For this review, take the finished solid that the model builds, in its own axes (mm). Round coordinates to 2 decimals unless told otherwise and drop trailing zeros. Write each loop counter-clockwise with the first axis right and the second up, starting at its lowest first coordinate (ties: lowest second). Pieces come first, ordered by that corner, then holes. Notation, with made-up numbers: M 6,-11.5 L 35,-11.5 A31 ccw 35,18.5 Z; hole C -28,-7.75 d1. An arc over 180 degrees is marked long. Answer in a Markdown table with one row per item.
```python
from build123d import *

# Parameters (mm, degrees)
SALIENTE_EXTRUIR1_DEPTH = 1
CROQUIS2_R              = 10
CORTAR_EXTRUIR1_DEPTH   = 57.577380639
CROQUIS3_R              = 1.5
CROQUIS3_R_2            = 2.5
CORTAR_EXTRUIR2_DEPTH   = 57.577380639
MATRIZC1_COUNT          = 4


with BuildPart() as part:
    # Croquis1 → Saliente-Extruir1 (new body)
    with BuildSketch(Plane.XY):
        with BuildLine():
            Line((-35, -40), (35, -40))
            ThreePointArc((35, -40), (38.535533906, -38.535533906), (40, -35))
            Line((40, -35), (40, 35))
            ThreePointArc((40, 35), (38.535533906, 38.535533906), (35, 40))
            Line((35, 40), (-35, 40))
            ThreePointArc((-35, 40), (-38.535533906, 38.535533906), (-40, 35))
            Line((-40, 35), (-40, -35))
            ThreePointArc((-40, -35), (-38.535533906, -38.535533906), (-35, -40))
        make_face()
    extrude(amount=SALIENTE_EXTRUIR1_DEPTH)

    # Croquis2 → Cortar-Extruir1 (cut, through all)
    with BuildSketch(Plane.XY.offset(1)):
        Circle(CROQUIS2_R)
        with BuildLine():
            Line((2.5, 16.770509831), (2.5, 30))
            ThreePointArc((2.5, 30), (3.232233047, 31.767766953), (5, 32.5))
            Line((5, 32.5), (22.928932188, 32.5))
            ThreePointArc((22.928932188, 32.5), (25.238631019, 30.956708581), (24.696699141, 28.232233047))
            Line((24.696699141, 28.232233047), (10.090774273, 13.626308179))
            ThreePointArc((10.090774273, 13.626308179), (8.683931275, 12.920265539), (7.134006274, 13.194921541))
            ThreePointArc((7.134006274, 13.194921541), (5.740251485, 13.858192988), (4.285714286, 14.374722712))
            ThreePointArc((4.285714286, 14.374722712), (2.995540686, 15.27647407), (2.5, 16.770509831))
        make_face()
        with BuildLine():
            Line((-10.090774273, 13.626308179), (-24.696699141, 28.232233047))
            ThreePointArc((-24.696699141, 28.232233047), (-25.238631019, 30.956708581), (-22.928932188, 32.5))
            Line((-22.928932188, 32.5), (-5, 32.5))
            ThreePointArc((-5, 32.5), (-3.232233047, 31.767766953), (-2.5, 30))
            Line((-2.5, 30), (-2.5, 16.770509831))
            ThreePointArc((-2.5, 16.770509831), (-2.995540686, 15.27647407), (-4.285714286, 14.374722712))
            ThreePointArc((-4.285714286, 14.374722712), (-5.740251485, 13.858192988), (-7.134006274, 13.194921541))
            ThreePointArc((-7.134006274, 13.194921541), (-8.683931275, 12.920265539), (-10.090774273, 13.626308179))
        make_face()
        with BuildLine():
            Line((32.5, 5), (32.5, 22.928932188))
            ThreePointArc((32.5, 22.928932188), (30.956708581, 25.238631019), (28.232233047, 24.696699141))
            Line((28.232233047, 24.696699141), (13.626308179, 10.090774273))
            ThreePointArc((13.626308179, 10.090774273), (12.920265539, 8.683931275), (13.194921541, 7.134006274))
            ThreePointArc((13.194921541, 7.134006274), (13.858192988, 5.740251485), (14.374722712, 4.285714286))
            ThreePointArc((14.374722712, 4.285714286), (15.27647407, 2.995540686), (16.770509831, 2.5))
            Line((16.770509831, 2.5), (30, 2.5))
            ThreePointArc((30, 2.5), (31.767766953, 3.232233047), (32.5, 5))
        make_face()
        with BuildLine():
            Line((16.770509831, -2.5), (30, -2.5))
            ThreePointArc((30, -2.5), (31.767766953, -3.232233047), (32.5, -5))
            Line((32.5, -5), (32.5, -22.928932188))
            ThreePointArc((32.5, -22.928932188), (30.956708581, -25.238631019), (28.232233047, -24.696699141))
            Line((28.232233047, -24.696699141), (13.626308179, -10.090774273))
            ThreePointArc((13.626308179, -10.090774273), (12.920265539, -8.683931275), (13.194921541, -7.134006274))
            ThreePointArc((13.194921541, -7.134006274), (13.858192988, -5.740251485), (14.374722712, -4.285714286))
            ThreePointArc((14.374722712, -4.285714286), (15.27647407, -2.995540686), (16.770509831, -2.5))
        make_face()
        with BuildLine():
            Line((5, -32.5), (22.928932188, -32.5))
            ThreePointArc((22.928932188, -32.5), (25.238631019, -30.956708581), (24.696699141, -28.232233047))
            Line((24.696699141, -28.232233047), (10.090774273, -13.626308179))
            ThreePointArc((10.090774273, -13.626308179), (8.683931275, -12.920265539), (7.134006274, -13.194921541))
            ThreePointArc((7.134006274, -13.194921541), (5.740251485, -13.858192988), (4.285714286, -14.374722712))
            ThreePointArc((4.285714286, -14.374722712), (2.995540686, -15.27647407), (2.5, -16.770509831))
            Line((2.5, -16.770509831), (2.5, -30))
            ThreePointArc((2.5, -30), (3.232233047, -31.767766953), (5, -32.5))
        make_face()
        with BuildLine():
            Line((-2.5, -16.770509831), (-2.5, -30))
            ThreePointArc((-2.5, -30), (-3.232233047, -31.767766953), (-5, -32.5))
            Line((-5, -32.5), (-22.928932188, -32.5))
            ThreePointArc((-22.928932188, -32.5), (-25.238631019, -30.956708581), (-24.696699141, -28.232233047))
            Line((-24.696699141, -28.232233047), (-10.090774273, -13.626308179))
            ThreePointArc((-10.090774273, -13.626308179), (-8.683931275, -12.920265539), (-7.134006274, -13.194921541))
            ThreePointArc((-7.134006274, -13.194921541), (-5.740251485, -13.858192988), (-4.285714286, -14.374722712))
            ThreePointArc((-4.285714286, -14.374722712), (-2.995540686, -15.27647407), (-2.5, -16.770509831))
        make_face()
        with BuildLine():
            Line((-32.5, -5), (-32.5, -22.928932188))
            ThreePointArc((-32.5, -22.928932188), (-30.956708581, -25.238631019), (-28.232233047, -24.696699141))
            Line((-28.232233047, -24.696699141), (-13.626308179, -10.090774273))
            ThreePointArc((-13.626308179, -10.090774273), (-12.920265539, -8.683931275), (-13.194921541, -7.134006274))
            ThreePointArc((-13.194921541, -7.134006274), (-13.858192988, -5.740251485), (-14.374722712, -4.285714286))
            ThreePointArc((-14.374722712, -4.285714286), (-15.27647407, -2.995540686), (-16.770509831, -2.5))
            Line((-16.770509831, -2.5), (-30, -2.5))
            ThreePointArc((-30, -2.5), (-31.767766953, -3.232233047), (-32.5, -5))
        make_face()
        with BuildLine():
            Line((-16.770509831, 2.5), (-30, 2.5))
            ThreePointArc((-30, 2.5), (-31.767766953, 3.232233047), (-32.5, 5))
            Line((-32.5, 5), (-32.5, 22.928932188))
            ThreePointArc((-32.5, 22.928932188), (-30.956708581, 25.238631019), (-28.232233047, 24.696699141))
            Line((-28.232233047, 24.696699141), (-13.626308179, 10.090774273))
            ThreePointArc((-13.626308179, 10.090774273), (-12.920265539, 8.683931275), (-13.194921541, 7.134006274))
            ThreePointArc((-13.194921541, 7.134006274), (-13.858192988, 5.740251485), (-14.374722712, 4.285714286))
            ThreePointArc((-14.374722712, 4.285714286), (-15.27647407, 2.995540686), (-16.770509831, 2.5))
        make_face()
    extrude(amount=-CORTAR_EXTRUIR1_DEPTH, mode=Mode.SUBTRACT)

    # Croquis3 → Cortar-Extruir2 (cut, through all)
    with BuildSketch(Plane.XY.offset(1)):
        with Locations((-36.25, 30)):
            Circle(CROQUIS3_R)
        with Locations((-36.25, 10)):
            Circle(CROQUIS3_R)
        with Locations((-36.25, -10)):
            Circle(CROQUIS3_R)
        with Locations((-36.25, -30)):
            Circle(CROQUIS3_R)
        with Locations(Location((36.25, -30, 0), (0, 0, 180))):
            Circle(CROQUIS3_R)
        with Locations(Location((36.25, -10, 0), (0, 0, 180))):
            Circle(CROQUIS3_R)
        with Locations(Location((36.25, 10, 0), (0, 0, 180))):
            Circle(CROQUIS3_R)
        with Locations(Location((36.25, 30, 0), (0, 0, 180))):
            Circle(CROQUIS3_R)
        with Locations((-36.25, 0)):
            Circle(CROQUIS3_R_2)
        with Locations(Location((36.25, 0, 0), (0, 0, 180))):
            Circle(CROQUIS3_R_2)
    cortar_extruir2 = extrude(amount=-CORTAR_EXTRUIR2_DEPTH, mode=Mode.SUBTRACT)

    # MatrizC1: Cortar-Extruir2 ×4 about axis
    matrizc1_axis = Axis((0, 0, 0), (0, 0, 1))
    for i in range(1, MATRIZC1_COUNT):
        add(cortar_extruir2.rotate(matrizc1_axis, i * 360 / MATRIZC1_COUNT), mode=Mode.SUBTRACT)


solid = part.part
```
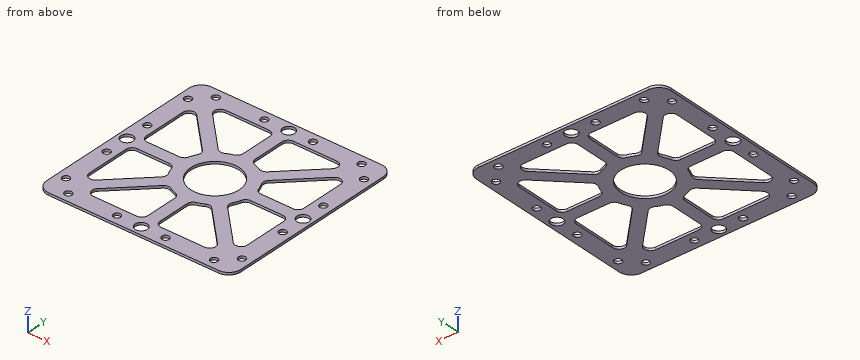
Q1. For probe 1 along Y at (x, z) = (-9, 0.95); probe 2 along X at (y, z) = (-0.5, 0.15); probe 3 along X at (y, z) = (18.5, 0.6), list the stretches that pass through material, from the lowest coordinate up.
Found:
| item | result |
|---|---|
| probe 1 | -40 to -37.37, -35.13 to -32.5, -12.99 to -4.36, 4.36 to 12.99, 32.5 to 35.13, 37.37 to 40 |
| probe 2 | -40 to -38.7, -33.8 to -9.99, 9.99 to 33.8, 38.7 to 40 |
| probe 3 | -40 to -32.5, -22.04 to -14.96, -2.5 to 2.5, 14.96 to 22.04, 32.5 to 40 |
Q2. Take a section at C-C (x = 20). State the section outline as (y, z) points, then the cut area to 3 significant figures.
Found:
| item | result |
|---|---|
| outline | M -40,0 L -32.5,0 L -32.5,1 L -40,1 Z; M -23.54,0 L -16.46,0 L -16.46,1 L -23.54,1 Z; M -2.5,0 L 2.5,0 L 2.5,1 L -2.5,1 Z; M 16.46,0 L 23.54,0 L 23.54,1 L 16.46,1 Z; M 32.5,0 L 40,0 L 40,1 L 32.5,1 Z |
| area | 34.1 mm² |
Q3. Take a section at D-D (y = 1.5). State the section outline as (x, z) points, then the cut area to 3 significant figures.
Found:
| item | result |
|---|---|
| outline | M -40,0 L -38.25,0 L -38.25,1 L -40,1 Z; M -34.25,0 L -9.89,0 L -9.89,1 L -34.25,1 Z; M 9.89,0 L 34.25,0 L 34.25,1 L 9.89,1 Z; M 38.25,0 L 40,0 L 40,1 L 38.25,1 Z |
| area | 52.2 mm² |
Q4. Take a section at A-A (y = -19.5). State the section outline as (x, z) points.
Found:
| item | result |
|---|---|
| outline | M -40,0 L -32.5,0 L -32.5,1 L -40,1 Z; M -23.04,0 L -15.96,0 L -15.96,1 L -23.04,1 Z; M -2.5,0 L 2.5,0 L 2.5,1 L -2.5,1 Z; M 15.96,0 L 23.04,0 L 23.04,1 L 15.96,1 Z; M 32.5,0 L 40,0 L 40,1 L 32.5,1 Z |
Q5. Take a section at B-B (y = 36.25). State the section outline as (x, z) points.
Found:
| item | result |
|---|---|
| outline | M -39.84,0 L -31.5,0 L -31.5,1 L -39.84,1 Z; M -28.5,0 L -11.5,0 L -11.5,1 L -28.5,1 Z; M -8.5,0 L -2.5,0 L -2.5,1 L -8.5,1 Z; M 2.5,0 L 8.5,0 L 8.5,1 L 2.5,1 Z; M 11.5,0 L 28.5,0 L 28.5,1 L 11.5,1 Z; M 31.5,0 L 39.84,0 L 39.84,1 L 31.5,1 Z |
Q6. Insertion check: P1, Ø1.8, axis at x = -36.25, y = -10, coming from the +Z side. The pin has a flat end and moves straight along its axis. Give the tip position at first contact, or say it passes through.
Found:
| item | result |
|---|---|
| P1 | through |
